Job drawing, mm, ordinate dimensions from the low corner. One solid piece. A direction names the side the tool comes from. Give positions to 0.01 mm unless a question says otherwise; leave off trailing zeros. Write each loop counter-clockwise with the first axis right and the second up, starting at its lowest first coordinate (ties: lowest second). Pieces come first, ordered by that corner, then holes. Notation, with made-up numbers: (73.5, 19) - (119.5, 19) arc R23 cw to (119.5, 42) - close; hole circle Ø2 at (35, 21.5). An arc over 180 degrees is marked (long way). Answer in a Markdown table with one row per item. Add a question column.
1. Probe line 1 along X through (y, z) = (10.5, 20); line 2 along X through (y, z) = (85.5, 71); line 3 along Y through (x, z) = (18, 100). List the from-to ranges inside material, lowest first.
2. Band-saw the part on D-D on x = 17. Write the cut outline in (y, z), plus the area to 3 significant figures.
3. Band-saw the part on A-A on z = 180. Write the cut outline in (x, y).
4. Which spindle directions (+Z, -Z, +X, -X, +Y, -Y) get a long thin tool onto all of the face, cutting with end or side? Do the marked faces 4, 5, 6, 7 and 8. Say none if no direction does.
5. Pull direction Y, two halves, no side cores. Call the marked faces 1, 2 and 3: released by +Y, released by -Y, zero draft, split by the parting line, or undercut.
6. Band-saw the part on B-B on x = 47. Write the cut outline in (y, z).
7. Band-saw the part on C-C on y = 31.5. Write the cut outline in (x, z).
8. Drop flat-ended pins along their axis: pin 1 Ø9 at (x, y) = (69, 56) entering from -Z; pin 2 Ø1 at (x, z) = (30, 129) entering from +Y; pin 3 Ø4 at (x, y) = (60, 44) entering from -Z; pin 4 Ø9 at (x, y) = (18.5, 67.5) entering from +Z. Give the stop position or say it passes through.
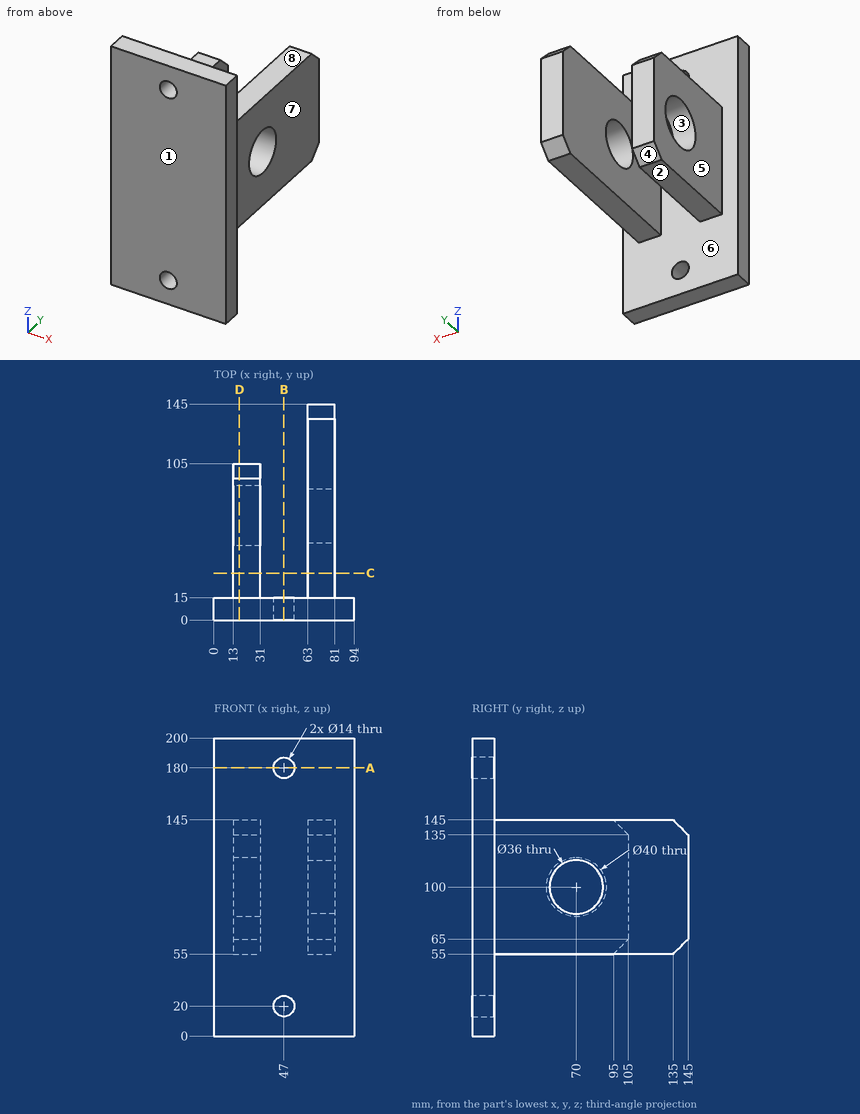
Values:
| question | item | result |
|---|---|---|
| 1 | line 1 | x = 0 to 40, 54 to 94 |
| 1 | line 2 | x = 13 to 31, 63 to 81 |
| 1 | line 3 | y = 0 to 50, 90 to 105 |
| 2 | outline | (0, 0) - (15, 0) - (15, 55) - (95, 55) - (105, 65) - (105, 135) - (95, 145) - (15, 145) - (15, 200) - (0, 200) - close; hole circle Ø40 at (70, 100) |
| 2 | area | 9,740 mm² |
| 3 | outline | (0, 0) - (40, 0) - (40, 15) - (0, 15) - close; (54, 0) - (94, 0) - (94, 15) - (54, 15) - close |
| 4 | face 4 | -Z, -X, +Y |
| 4 | face 5 | +Z, -Z, -X, +Y |
| 4 | face 6 | +Y |
| 4 | face 7 | +Z, -Z, +X, +Y |
| 4 | face 8 | +Z, +X, -X, +Y |
| 5 | face 1 | released by -Y |
| 5 | face 2 | zero draft |
| 5 | face 3 | undercut |
| 6 | outline | (0, 0) - (15, 0) - (15, 13) - (0, 13) - close; (0, 27) - (15, 27) - (15, 173) - (0, 173) - close; (0, 187) - (15, 187) - (15, 200) - (0, 200) - close |
| 7 | outline | (13, 55) - (31, 55) - (31, 145) - (13, 145) - close; (63, 55) - (81, 55) - (81, 145) - (63, 145) - close |
| 8 | pin 1 | stops at z = 55 |
| 8 | pin 2 | stops at y = 105 |
| 8 | pin 3 | passes through |
| 8 | pin 4 | stops at z = 145 |
